Geometry: final body of the model. Coordinates: model frame, mm. Coordinates: 2 decimals unless noted, no trailing zeros. Loops run counter-clockwise (first coordinate to the right, second up) from the corner with the lowest first, then second, coordinate; pieces in that order, holes last. Notation, with made-up numbers: (39, 66.25) - (92, 66.25) arc R7 cw to (92, 76.25) - close; hole circle Ø6 at (14.5, 37). An arc over 180 degrees is marked (long way). Answer in a Markdown table with one row per item.
from build123d import *

# Parameters (mm, degrees)
SZKIC1_R                    = 49
DODANIE_WYCI_GNI_CIE1_DEPTH = 2
WYTNIJ_WYCI_GNI_CIE2_REACH  = 4
SZKIC4_R                    = 3.5
OTW_R_POD_RUB_M21_D         = 2.6
OTW_R_POD_RUB_M21_DEPTH     = 2
OTW_R_POD_RUB_M22_D         = 2.6
OTW_R_POD_RUB_M22_DEPTH     = 2


with BuildPart() as part:
    # Szkic1 → Dodanie-wyciągnięcie1 (new body)
    with BuildSketch(Plane.XY):
        Circle(SZKIC1_R)
    extrude(amount=DODANIE_WYCI_GNI_CIE1_DEPTH)

    # Szkic4 → Wytnij-wyciągnięcie2 (cut, up to next)
    with BuildSketch(Plane(origin=(0, 0, 0), x_dir=(-1, 0, 0), z_dir=(0, 0, -1)), mode=Mode.PRIVATE) as wytnij_wyci_gni_cie2_sk1:
        Circle(SZKIC4_R)
    wytnij_wyci_gni_cie2_tool1 = extrude(wytnij_wyci_gni_cie2_sk1.sketch, amount=-WYTNIJ_WYCI_GNI_CIE2_REACH, mode=Mode.PRIVATE) & part.part
    add(wytnij_wyci_gni_cie2_tool1.solids().sort_by_distance((0, 0, 0))[0], mode=Mode.SUBTRACT)

    # Otwór pod śrubę M21
    with Locations(Plane(origin=(-17.5, 7.5, 0), x_dir=(-1, 0, 0), z_dir=(0, 0, -1))):
        with Locations((0, 0), (0, -15), (-35, -15), (-35, 0)):
            Hole(OTW_R_POD_RUB_M21_D / 2, depth=OTW_R_POD_RUB_M21_DEPTH)

    # Otwór pod śrubę M22
    with Locations(Plane(origin=(-7.1, 0, 0), x_dir=(-1, 0, 0), z_dir=(0, 0, -1))):
        with Locations((0, 0), (-14.2, 0)):
            Hole(OTW_R_POD_RUB_M22_D / 2, depth=OTW_R_POD_RUB_M22_DEPTH)


solid = part.part
(1) Cut plane A-A on x = 0. Output: boundary loops of the cut face in (y, z), then the cut area to 3 significant figures.
Verdict:
| item | result |
|---|---|
| outline | (-49, 0) - (-3.5, 0) - (-3.5, 2) - (-49, 2) - close; (3.5, 0) - (49, 0) - (49, 2) - (3.5, 2) - close |
| area | 182 mm² |
(2) Cut plane B-B on y = 0. Output: boundary loops of the cut face in (x, z), then the cut area to 3 significant figures.
Verdict:
| item | result |
|---|---|
| outline | (-49, 0) - (-8.4, 0) - (-8.4, 2) - (-49, 2) - close; (-5.8, 0) - (-3.5, 0) - (-3.5, 2) - (-5.8, 2) - close; (3.5, 0) - (5.8, 0) - (5.8, 2) - (3.5, 2) - close; (8.4, 0) - (49, 0) - (49, 2) - (8.4, 2) - close |
| area | 172 mm² |
(3) Cut plane D-D on x = 42.5. Output: boundary loops of the cut face in (y, z), then the cut area to 4 significant figures.
Verdict:
| item | result |
|---|---|
| outline | (-24.39, 0) - (24.39, 0) - (24.39, 2) - (-24.39, 2) - close |
| area | 97.55 mm² |
(4) Cut plane C-C on z = 0.3. Output: boundary loops of the cut face in (x, y), then the cut area to 3 significant figures.
Verdict:
| item | result |
|---|---|
| outline | circle Ø98 at (0, 0); hole circle Ø2.6 at (-17.5, -7.5); hole circle Ø2.6 at (-17.5, 7.5); hole circle Ø2.6 at (-7.1, 0); hole circle Ø7 at (0, 0); hole circle Ø2.6 at (7.1, 0); hole circle Ø2.6 at (17.5, -7.5); hole circle Ø2.6 at (17.5, 7.5) |
| area | 7,470 mm² |
(5) First-contact query: pin 1 Ø2 at (x, y) = (-7.1, 0) entering from +Z; pin 2 Ø1 at (x, z) = (18, 1.5) entering from -Y; pin 3 Ø1 at (x, z) = (29, 1.5) entering from +Y. Flat tips, straight axial feed; report the tip coordinate or a pass-through.
Verdict:
| item | result |
|---|---|
| pin 1 | passes through |
| pin 2 | stops at y = -45.77 |
| pin 3 | stops at y = 39.86 |
(6) Ray query, probe 1 along Y at (x, z) = (-17.5, 0.7); probe 2 along Y at (x, z) = (20.5, 1.05); probe 3 along Y at (x, z) = (19.5, 1.1). Return the intervals inside material, ascending.
Verdict:
| item | result |
|---|---|
| probe 1 | y = -45.77 to -8.8, -6.2 to 6.2, 8.8 to 45.77 |
| probe 2 | y = -44.51 to 44.51 |
| probe 3 | y = -44.95 to 44.95 |
